Check sheet for the modelled part. Datum: model origin and axes. Units: mm. Coordinates: 2 decimals unless noted, no trailing zeros. Order: outer loops, then holes, each group sorted by start corner. A loop starts at its lowest first (then second) coordinate and runs counter-clockwise, first axis right, second up.
1. Cross-section at A-A (y = -15.6). Enter the section's corners in (x, z).
2. Thickness scan on line 1 (Y direction, x = -2.95, z = 0.3); line 2 (X direction, y = 6, z = 0.9); line 3 (Y direction, x = -13, z = 0.7). Record the ranges inside material, lowest first.
3. Draft check along X on faces 1 (the cylindrical face through (20.255, -14.113, 0.493)), 2 (the flat face through (-6, 1, 1)). Enter one of: released by +X, released by -X, zero draft, split by the parting line, or undercut.
4. Cross-section at B-B (x = 20.45). Enter the section's corners in (y, z), then the cut area to 3 significant figures.
5. Cross-section at D-D (x = -14.5). Enter the section's corners in (y, z), then the cut area to 3 significant figures.
6. Gauge pin test, flat end, axial feed: pin 1 Ø2.5 at (x, y) = (-2.95, 5.2) entering from +Z. Record the tip position at first contact, or that the pin passes through.
7. Cross-section at C-C (z = 0.85). Count the separate pieces of the cut face and the enclosed holes in it, then the cut area to 3 significant figures.
```python
from build123d import *

# Parameters (mm, degrees)
SKETCH_1_R      = 1.5
EXTRUDE_1_DEPTH = 1


with BuildPart() as part:
    # Эскиз1 → Бобышка-Вытянуть1 (new body)
    with BuildSketch(Plane.XY):
        Polygon((-23.75, 46), (-23.75, -46), (-8.75, -46), (-8.75, -21), (23.75, -21), (23.75, 21), (-8.75, 21), (-8.75, 46), align=None)
        with Locations((-13.986702311, 30.5)):
            Circle(SKETCH_1_R, mode=Mode.SUBTRACT)
        with Locations((-13.986702311, -30.5)):
            Circle(SKETCH_1_R, mode=Mode.SUBTRACT)
        with Locations((-2.95, -15.6)):
            Circle(SKETCH_1_R, mode=Mode.SUBTRACT)
        with Locations((-2.95, -5.2)):
            Circle(SKETCH_1_R, mode=Mode.SUBTRACT)
        with Locations((-2.95, 5.2)):
            Circle(SKETCH_1_R, mode=Mode.SUBTRACT)
        with Locations((-2.95, 15.6)):
            Circle(SKETCH_1_R, mode=Mode.SUBTRACT)
        with Locations((20.45, 15.6)):
            Circle(SKETCH_1_R, mode=Mode.SUBTRACT)
        with Locations((20.45, 5.2)):
            Circle(SKETCH_1_R, mode=Mode.SUBTRACT)
        with Locations((20.45, -5.2)):
            Circle(SKETCH_1_R, mode=Mode.SUBTRACT)
        with Locations((20.45, -15.6)):
            Circle(SKETCH_1_R, mode=Mode.SUBTRACT)
    extrude(amount=EXTRUDE_1_DEPTH)


solid = part.part
```
Data:
1. outline: (-23.75, 0) - (-4.45, 0) - (-4.45, 1) - (-23.75, 1) - close; (-1.45, 0) - (18.95, 0) - (18.95, 1) - (-1.45, 1) - close; (21.95, 0) - (23.75, 0) - (23.75, 1) - (21.95, 1) - close
2. line 1: y = -21 to -17.1, -14.1 to -6.7, -3.7 to 3.7, 6.7 to 14.1, 17.1 to 21
2. line 2: x = -23.75 to -4.22, -1.68 to 19.18, 21.72 to 23.75
2. line 3: y = -46 to -31.63, -29.37 to 29.37, 31.63 to 46
3. face 1: undercut
3. face 2: zero draft
4. outline: (-21, 0) - (-17.1, 0) - (-17.1, 1) - (-21, 1) - close; (-14.1, 0) - (-6.7, 0) - (-6.7, 1) - (-14.1, 1) - close; (-3.7, 0) - (3.7, 0) - (3.7, 1) - (-3.7, 1) - close; (6.7, 0) - (14.1, 0) - (14.1, 1) - (6.7, 1) - close; (17.1, 0) - (21, 0) - (21, 1) - (17.1, 1) - close
4. area: 30.0 mm2
5. outline: (-46, 0) - (-31.91, 0) - (-31.91, 1) - (-46, 1) - close; (-29.09, 0) - (29.09, 0) - (29.09, 1) - (-29.09, 1) - close; (31.91, 0) - (46, 0) - (46, 1) - (31.91, 1) - close
5. area: 86.4 mm2
6. pin 1: passes through
7. separate pieces: 1
7. enclosed holes: 10
7. area: 2,670 mm2
